Can you work these out from the model? Positions are in its coordinate system, mm. Face numbers are marked on the shaded views. A direction names the side the tool comes from. Give positions to 0.01 mm unless a question says otherwise; leave off trailing zeros. Order: outer loops, then holes, each group sorted by start corner. A loop starts at its lowest first (then second) coordinate and runs counter-clockwise, first axis right, second up. Notation, with made-up numbers: (51.25, 75) - (108.25, 75) arc R18 ccw to (108.25, 88) - close; hole circle Ø10 at (50.25, 21.5). An arc over 180 degrees is marked (long way). One line per question, with ' | ' between items.
```python
from build123d import *

# Parameters (mm, degrees)
SKETCH1_R              = 2.25
BASE_FLANGE1_DEPTH     = 1.5748
SKETCHED_START         = -31.998080115
SKETCHED_BEND1_DEPTH   = 63.99616023
SKETCHED_BEND1_2_DEPTH = 63.99616023


# Read off the part's stored shape, not the designer's step: Sketched Bend1
# Sheet-metal steps are written as plain solids
with BuildPart() as part:
    # Sketch1 → Base-Flange1 (new body)
    with BuildSketch(Plane.XY):
        with BuildLine():
            Line((0.25, 38.499188303), (0.25, 26.248809497))
            ThreePointArc((0.25, 26.248809497), (26.498809497, 0), (0.25, -26.248809497))
            Line((0.25, -26.248809497), (0.25, -38.499188303))
            ThreePointArc((0.25, -38.499188303), (11.317914827, -36.837266048), (21.409644298, -31.998080115))
            Line((21.409644298, -31.998080115), (102.929679939, -31.998080115))
            Line((102.929679939, -31.998080115), (196.443018387, -31.998080115))
            Line((196.443018387, -31.998080115), (196.443018387, 31.998080115))
            Line((196.443018387, 31.998080115), (102.929679939, 31.998080115))
            Line((102.929679939, 31.998080115), (21.409644298, 31.998080115))
            ThreePointArc((21.409644298, 31.998080115), (11.317914827, 36.837266048), (0.25, 38.499188303))
        make_face()
        with Locations((12.819894984, 30.949964339)):
            Circle(SKETCH1_R, mode=Mode.SUBTRACT)
        with Locations((30.949964339, 12.819894984)):
            Circle(SKETCH1_R, mode=Mode.SUBTRACT)
        with Locations((30.949964339, -12.819894984)):
            Circle(SKETCH1_R, mode=Mode.SUBTRACT)
        with Locations((12.819894984, -30.949964339)):
            Circle(SKETCH1_R, mode=Mode.SUBTRACT)
    extrude(amount=-BASE_FLANGE1_DEPTH)

    # Sketched Bend1 outline → Sketched Bend1 (cut)
    with BuildSketch(Plane(origin=(0, 0, 0), x_dir=(1, 0, 0), z_dir=(0, 1, 0)).offset(SKETCHED_START)):
        with BuildLine():
            ThreePointArc((107.11495185, 1.5748), (108.71495025, 1.153848498), (109.90062672, 0))
            Line((109.90062672, 0), (196.443018387, 0))
            Line((196.443018387, 0), (196.443018387, 1.5748))
            Line((196.443018387, 1.5748), (107.11495185, 1.5748))
        make_face()
    extrude(amount=SKETCHED_BEND1_DEPTH, mode=Mode.SUBTRACT)

    # Sketched Bend1 2 outline → Sketched Bend1 2 (add)
    with BuildSketch(Plane(origin=(0, 0, 0), x_dir=(1, 0, 0), z_dir=(0, 1, 0)).offset(SKETCHED_START)):
        with BuildLine():
            Line((108.79135185, -1.6764), (108.79135185, -87.381707553))
            Line((108.79135185, -87.381707553), (110.36615185, -87.381707553))
            Line((110.36615185, -87.381707553), (110.36615185, -1.6764))
            ThreePointArc((110.36615185, -1.6764), (110.247609474, -0.806481813), (109.90062672, 0))
            Line((109.90062672, 0), (107.11495185, 0))
            ThreePointArc((107.11495185, 0), (108.300345658, -0.491006192), (108.79135185, -1.6764))
        make_face()
    extrude(amount=SKETCHED_BEND1_2_DEPTH)


solid = part.part
```
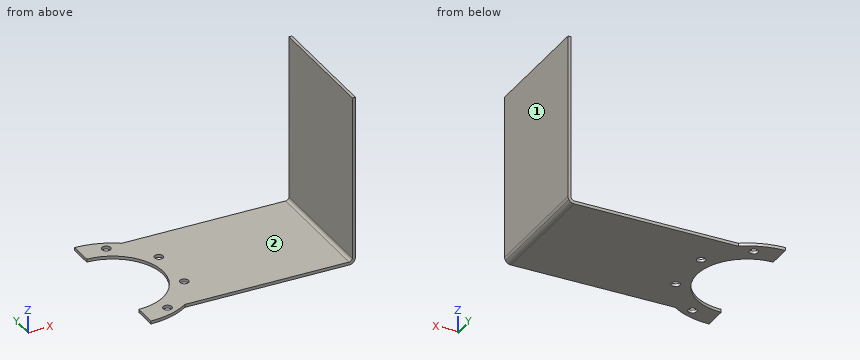
(1) On a 3-axis mill with a long thin cutter (end or side, diameter ignored), from which of +Z, -Z, +X, -X, +Y, -Y can I reach the whole of each face in a straight line? I mean the marked faces 1 and 2. Say none if no direction works.
Answer below:
face 1: +Z, -Z, +X, +Y, -Y | face 2: +Z, -X, +Y, -Y
(2) Will these pins go through, and if not, where does the flat tip stop? pin 1 (4 mm diameter, centred on x = 12.82, y = 30.95, fed in from +Z); pin 2 (6 mm diameter, centred on y = 19.5, z = 32, fed in from -X).
Answer below:
pin 1: through | pin 2: x = 108.79
(3) If I drill on line 1 (Z direction, x = 65.5, y = 10.5); line 2 (X direction, y = 31, z = 55.5), over which ranges is the centre line in solid material (lowest first)?
Answer below:
line 1: -1.57 to 0 | line 2: 108.79 to 110.37
(4) Imagine slicing it at A-A (x = 16.5). List the corners of the cut face in (y, z) for me, and give its area (3 significant figures).
Answer below:
outline: (-34.82, -1.57) - (-20.61, -1.57) - (-20.61, 0) - (-34.82, 0) - close; (20.61, -1.57) - (34.82, -1.57) - (34.82, 0) - (20.61, 0) - close | area: 44.7 mm^2
(5) Imagine slicing it at D-D (y = 0). List the corners of the cut face in (x, z) for me.
Answer below:
outline: (26.5, -1.57) - (107.11, -1.57) arc R3.25 ccw to (110.37, 1.68) - (110.37, 87.38) - (108.79, 87.38) - (108.79, 1.68) arc R1.68 cw to (107.11, 0) - (26.5, 0) - close
(6) Imagine slicing it at B-B (y = -17). List the corners of the cut face in (x, z) for me, and give its area (3 significant figures).
Answer below:
outline: (20.25, -1.57) - (107.11, -1.57) arc R3.25 ccw to (110.37, 1.68) - (110.37, 87.38) - (108.79, 87.38) - (108.79, 1.68) arc R1.68 cw to (107.11, 0) - (20.25, 0) - close | area: 278 mm^2
(7) Imagine slicing it at C-C (z = 10). List the corners of the cut face in (x, y) for me.
Answer below:
outline: (108.79, -32) - (110.37, -32) - (110.37, 32) - (108.79, 32) - close
